```python
from build123d import *

# Parameters (mm, degrees)
F0_R     = 3.1
F0_R_2   = 1.26
F1_DEPTH = 5
F2_SIZE2 = 0.5196152423
F2_SIZE  = 0.3
F3_SCALE = 3


with BuildPart() as f1:
    # F0 (on Top) → F1 (new body)
    with BuildSketch(Plane.XY):
        Circle(F0_R)
        Circle(F0_R_2, mode=Mode.SUBTRACT)
    extrude(amount=F1_DEPTH)

    # F2
    f2_edges = [f1.edges().sort_by_distance(p)[0] for p in [
        (-1.26, 0, 5),
    ]]
    f2_side = f1.faces().sort_by_distance((-3.012319, 0, 5))[0]
    chamfer(f2_edges, length=F2_SIZE, length2=F2_SIZE2, reference=f2_side)


with BuildPart() as f1_1:
    # F3: moved
    add(f1.part.scale(F3_SCALE))


solid = f1_1.part
```
Geometry: final body of the model. Coordinates: model frame, mm. Coordinates: 2 decimals unless noted, no trailing zeros. Write each loop counter-clockwise with the first axis right and the second up, starting at its lowest first coordinate (ties: lowest second). Pieces come first, ordered by that corner, then holes. Notation, with made-up numbers: M 85.25,-7.5 L 144.25,-7.5 A11 ccw 144.25,2.5 Z; hole C 56.25,27 d11. An arc over 180 degrees is marked long. Answer as CSV lines item,"result". Start each with the question number.
Q1. Cut plane A-A on y = 0. Return the cut outline in (x, z).
Q2. Pin query (flat end, axial travel): P1, Ø8, axis at x = 5, z = 10, coming from the +Y side; P2, Ø7, axis at x = 0, y = 0, coming from the +Z side; P3, Ø5, axis at x = -4, z = 7.5, coming from the -Y side; P4, Ø1.5, axis at x = 3.5, z = 12.5, coming from the +Y side. Return the tip coordinate at first contact, or that it passes through.
Q3. Line query: line 1 (Y direction, x = 0, z = 9.25); line 2 (X direction, y = 0.25, z = 2.75); line 3 (X direction, y = 1.25, z = 8.75). Output: solid intervals per line, ascending. Write a range as from..to.
Q4. Cut plane C-C on z = 10. Return the cut outline in (x, y), then the cut area to 3 significant figures.
Q5. Cut plane D-D on x = 7. Return the cut outline in (y, z), then the cut area to 3 significant figures.
Q6. Mould query, pull axis Y, two halves, no side actions, for faces 1 (the cylindrical face through (-0.82, -3.69, 6.63)), 2 (the flat face through (4, 0, 0)), 3 (the cylindrical face through (5, 7.84, 7.4)). Classes: released by +Y, released by -Y, zero draft, split by the parting line, or undercut.
Findings below:
1,outline,"M -9.3,0 L -3.78,0 L -3.78,13.44 L -4.68,15 L -9.3,15 Z; M 3.78,0 L 9.3,0 L 9.3,15 L 4.68,15 L 3.78,13.44 Z"
2,P1,"stops at y = 9.25"
2,P2,"passes through"
2,P3,"stops at y = -9.18"
2,P4,"stops at y = 8.88"
3,line 1,"y = -9.3..-3.78, 3.78..9.3"
3,line 2,"x = -9.3..-3.77, 3.77..9.3"
3,line 3,"x = -9.22..-3.57, 3.57..9.22"
4,outline,"C 0,0 d18.6; hole C 0,0 d7.56"
4,area,"227 mm2"
5,outline,"M -6.12,0 L 6.12,0 L 6.12,15 L -6.12,15 Z"
5,area,"184 mm2"
6,face 1,"undercut"
6,face 2,"zero draft"
6,face 3,"split by the parting line"
